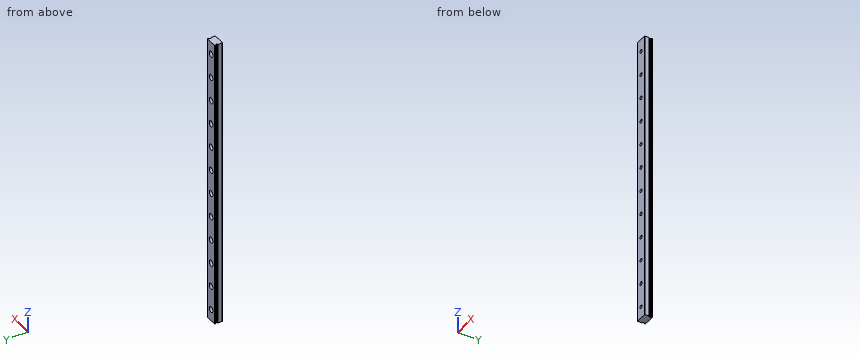
```python
from build123d import *

# Parameters (mm, degrees)
EXTRUDE_1_DEPTH        = 300
SKETCH_2_R             = 3
SKETCH_2_R_2           = 1.75
CUT_EXTRUDE_1_DEPTH    = 4.5
SKETCH_2_2_R           = 1.75
CUT_EXTRUDE_2_DEPTH    = 9
PATTERN_LINEAR_1_COUNT = 16
PATTERN_LINEAR_1_PITCH = 25


with BuildPart() as part:
    # Эскиз1 → Бобышка-Вытянуть1 (new body)
    with BuildSketch(Plane.XY):
        with BuildLine():
            Line((-6, 3.7), (-5.7, 4))
            Line((-5.7, 4), (5.7, 4))
            Line((5.7, 4), (6, 3.7))
            Line((6, 3.7), (6, 2.451013544))
            ThreePointArc((6, 2.451013544), (5.597935912, 2.202976267), (5.354599002, 1.798050138))
            Line((5.354599002, 1.798050138), (4.643514056, 1.798050138))
            Line((4.643514056, 1.798050138), (4.643514056, 1.201949862))
            Line((4.643514056, 1.201949862), (5.354599002, 1.201949862))
            ThreePointArc((5.354599002, 1.201949862), (5.597935912, 0.797023733), (6, 0.548986456))
            Line((6, 0.548986456), (6, -3.7))
            Line((6, -3.7), (5.7, -4))
            Line((5.7, -4), (-5.7, -4))
            Line((-5.7, -4), (-6, -3.7))
            Line((-6, -3.7), (-6, 0.548986456))
            ThreePointArc((-6, 0.548986456), (-5.597935912, 0.797023733), (-5.354599002, 1.201949862))
            Line((-5.354599002, 1.201949862), (-4.643514056, 1.201949862))
            Line((-4.643514056, 1.201949862), (-4.643514056, 1.798050138))
            Line((-4.643514056, 1.798050138), (-5.354599002, 1.798050138))
            ThreePointArc((-5.354599002, 1.798050138), (-5.597935912, 2.202976267), (-6, 2.451013544))
            Line((-6, 2.451013544), (-6, 3.7))
        make_face()
    extrude(amount=EXTRUDE_1_DEPTH)

    # Эскиз2 → Вырез-Вытянуть1 (cut)
    with BuildSketch(Plane(origin=(0, 4, 0), x_dir=(1, 0, 0), z_dir=(0, 1, 0))):
        with Locations((0, -12)):
            Circle(SKETCH_2_R)
        with Locations((0, -12)):
            Circle(SKETCH_2_R_2, mode=Mode.SUBTRACT)
    cut_extrude_1 = extrude(amount=-CUT_EXTRUDE_1_DEPTH, mode=Mode.SUBTRACT)

    # Эскиз2<2> → Вырез-Вытянуть2 (cut, through all)
    with BuildSketch(Plane(origin=(0, 4, 0), x_dir=(1, 0, 0), z_dir=(0, 1, 0))):
        with Locations((0, -12)):
            Circle(SKETCH_2_2_R)
    cut_extrude_2 = extrude(amount=-CUT_EXTRUDE_2_DEPTH, mode=Mode.SUBTRACT)

    # Линейный массив1: Вырез-Вытянуть1, Вырез-Вытянуть2 ×16
    with Locations(*[(0, 0, i * PATTERN_LINEAR_1_PITCH) for i in range(1, PATTERN_LINEAR_1_COUNT)]):
        add(cut_extrude_1, mode=Mode.SUBTRACT)
        add(cut_extrude_2, mode=Mode.SUBTRACT)


solid = part.part
```
Source: CAD feature listing. Evaluate the final solid. Frame: model axes, mm. Give positions to 0.01 mm unless a question says otherwise; leave off trailing zeros. Order: outer loops, then holes, each group sorted by start corner. A loop starts at its lowest first (then second) coordinate and runs counter-clockwise, first axis right, second up.
(1) Material intervals for line 1 along Y through (x, z) = (-5, 210.5); line 2 along X through (y, z) = (2.75, 212.5); line 3 along X through (y, z) = (-2.25, 62), sorted ascending.
(2) Contact query for flat-ended pins moving along their axis: P1, Ø4.5, axis at x = 0, z = 112, coming from the +Y side; P2, Ø4.5, axis at x = 0, z = 37, coming from the -Y side. Output: stop coordinate, or through.
(3) Section query A-A (z = 279.5). Return the cut outline in (x, y).
Outcome:
1. line 1: y = -4 to 1.2, 1.8 to 4
1. line 2: x = -6 to -2.96, 2.96 to 6
1. line 3: x = -6 to -1.75, 1.75 to 6
2. P1: stops at y = -0.5
2. P2: stops at y = -4
3. outline: (-6, -3.7) - (-5.7, -4) - (5.7, -4) - (6, -3.7) - (6, 0.55) arc R1 cw to (5.35, 1.2) - (4.64, 1.2) - (4.64, 1.8) - (5.35, 1.8) arc R1 cw to (6, 2.45) - (6, 3.7) - (5.7, 4) - (-5.7, 4) - (-6, 3.7) - (-6, 2.45) arc R1 cw to (-5.35, 1.8) - (-4.64, 1.8) - (-4.64, 1.2) - (-5.35, 1.2) arc R1 cw to (-6, 0.55) - close
